Build history of the part. All positions in model axes, mm. A direction names the side the tool comes from. Round coordinates to 2 decimals unless told otherwise and drop trailing zeros. Order: outer loops, then holes, each group sorted by start corner. A loop starts at its lowest first (then second) coordinate and runs counter-clockwise, first axis right, second up. Notation, with made-up numbers: M 70.5,25 L 123.5,25 A22 ccw 123.5,62 Z; hole C 17,86 d9. An arc over 180 degrees is marked long. One line per item, written item: value. Start each with the question number.
Item 1: Pin check, flat tips, straight feed: pin 1 (5 mm diameter, centred on y = 7.5, z = 7.5, fed in from +X); pin 2 (1 mm diameter, centred on x = 14.5, y = 5.5, fed in from +Z); pin 3 (1.5 mm diameter, centred on x = 3.5, y = 3, fed in from +Z). Stop position of each tip, or through.
Item 2: Band-saw the part on B-B, the plane y = 4.25. Write the cut outline in (x, z), then the cut area to 3 significant figures.
Item 3: Band-saw the part on A-A, the plane z = 6.75. Write the cut outline in (x, y), then the cut area to 3 significant figures.
Item 4: Band-saw the part on D-D, the plane y = 8.5. Write the cut outline in (x, z).
Item 5: Tool access for faces 5 (the flat face through (8, 13, 5)), 6 (the flat face through (16, 8, 5)), 7 (the flat face through (11.46, 8.11, 21.61)): list every direction of +Z, -Z, +X, -X, +Y, -Y with a clear straight run to the whole face (end or side of a thin tool).
Item 6: Band-saw the part on C-C, the plane z = 12. Write the cut outline in (x, y).
Item 7: Two-plate mould, pull along Y, no slides. Class faces 1 (the flat face through (6, 0, 10)), 2 (the flat face through (8, 8, 10)), 3 (the flat face through (6, 16, 10)), 4 (the flat face through (0, 8, 13)): +Y half, -Y half, draft (parallel to the pull), parting line (faces both ways), or undercut.
Item 8: Probe L1, parallel to X at y = 11.5, z = 9; L2, parallel to X at y = 14, z = 8.25. List the from-to ranges inside material, lowest first.
```python
from build123d import *

# Parameters (mm, degrees)
SKETCH_1_W      = 16
SKETCH_1_H      = 16
SKETCH_1_W_2    = 10
SKETCH_1_H_2    = 10
EXTRUDE_1_DEPTH = 10
EXTRUDE_2_DEPTH = 16
EXTRUDE_3_DEPTH = 5


with BuildPart() as part:
    # 草图1 → 凸台-拉伸1 (new body)
    with BuildSketch(Plane.XY):
        with Locations((8, 8)):
            Rectangle(SKETCH_1_W, SKETCH_1_H)
        with Locations((8, 8)):
            Rectangle(SKETCH_1_W_2, SKETCH_1_H_2, mode=Mode.SUBTRACT)
    extrude(amount=EXTRUDE_1_DEPTH)

    # 草图2 → 凸台-拉伸2 (add)
    with BuildSketch(Plane.XZ):
        Polygon((0, 10), (0, 26), (16, 10), align=None)
    extrude(amount=-EXTRUDE_2_DEPTH)

    # 草图6 → 凸台-拉伸3 (add)
    with BuildSketch(Plane(origin=(13, 0, 13), x_dir=(0.7071067811865475, 0, -0.7071067811865477), z_dir=(0.7071067811865477, 0, 0.7071067811865475))):
        with BuildLine():
            ThreePointArc((-7.071067812, 16), (-15.071067812, 8), (-7.071067812, 0))
            Line((-7.071067812, 0), (-7.071067812, 16))
        make_face()
        with BuildLine():
            Line((-7.071067812, 16), (-7.071067812, 0))
            ThreePointArc((-7.071067812, 0), (-1.414213562, 2.343145751), (0.928932188, 8))
            ThreePointArc((0.928932188, 8), (-1.414213562, 13.656854249), (-7.071067812, 16))
        make_face()
    extrude(amount=EXTRUDE_3_DEPTH)


solid = part.part
```
Output:
1. pin 1: stops at x = 16
1. pin 2: stops at z = 19.07
1. pin 3: stops at z = 23.41
2. outline: M 0,0 L 3,0 L 3,10 L 13,10 L 13,0 L 16,0 L 16,10 L 13,13 L 16.53,16.54 L 6.54,26.53 L 3,23 L 0,26 Z
2. area: 259 mm²
3. outline: M 0,0 L 16,0 L 16,16 L 0,16 Z; hole M 3,3 L 13,3 L 13,13 L 3,13 Z
3. area: 156 mm²
4. outline: M 0,0 L 3,0 L 3,10 L 13,10 L 13,0 L 16,0 L 16,10 L 13.65,12.35 L 17.18,15.89 L 5.89,27.18 L 2.35,23.65 L 0,26 Z
5. face 5: -Z
5. face 6: -Z, +X, +Y, -Y
5. face 7: +Z, +X, +Y, -Y
6. outline: M 0,0 L 14,0 L 14,16 L 0,16 Z
7. face 1: -Y half
7. face 2: undercut
7. face 3: +Y half
7. face 4: draft
8. L1: x = 0 to 3, 13 to 16
8. L2: x = 0 to 16
